```python
from build123d import *

# Parameters (mm, degrees)
SKETCH1_W           = 30
SKETCH1_H           = 19.61
SKETCH1_R           = 2.25
BOSS_EXTRUDE1_DEPTH = 7
SKETCH2_R           = 3.6
CUT_EXTRUDE1_DEPTH  = 2.8
FILLET2_R           = 5
BOSS_EXTRUDE2_DEPTH = 30


with BuildPart() as part:
    # Sketch1 → Boss-Extrude1 (new body)
    with BuildSketch(Plane.XY):
        Rectangle(SKETCH1_W, SKETCH1_H)
        with Locations((-10, -3.805)):
            Circle(SKETCH1_R, mode=Mode.SUBTRACT)
        with Locations((10, -3.805)):
            Circle(SKETCH1_R, mode=Mode.SUBTRACT)
    extrude(amount=BOSS_EXTRUDE1_DEPTH)

    # Sketch2 → Cut-Extrude1 (cut)
    with BuildSketch(Plane.XY.offset(7)):
        with Locations((-10, -3.805)):
            Circle(SKETCH2_R)
        with Locations((10, -3.805)):
            Circle(SKETCH2_R)
    extrude(amount=-CUT_EXTRUDE1_DEPTH, mode=Mode.SUBTRACT)

    # Fillet2
    fillet2_edges = [part.edges().sort_by_distance(p)[0] for p in [
        (15, -9.805, 3.5),
        (-15, -9.805, 3.5),
    ]]
    fillet(fillet2_edges, radius=FILLET2_R)

    # Sketch3 → Boss-Extrude2 (add, through all)
    with BuildSketch(Plane.ZY.offset(15)):
        Polygon((7, 1.805), (7, 9.805), (19, 9.805), (19, 6.805), align=None)
    extrude(amount=-BOSS_EXTRUDE2_DEPTH)


solid = part.part
```
Part model, mm, in its own coordinate system. A direction names the side the tool comes from. Round coordinates to 2 decimals unless told otherwise and drop trailing zeros. Loops run counter-clockwise (first coordinate to the right, second up) from the corner with the lowest first, then second, coordinate; pieces in that order, holes last.
Item 1: Cut at D-D, the plane x = 4.5. Give the cut face in (y, z) (3 decimals).
Item 2: Cut at A-A, the plane x = 9. Give the cut face in (y, z) (3 decimals), then the cut area to 3 significant figures.
Item 3: Cut at C-C, the plane y = -2.75. Give the cut face in (x, z), then the cut area to 3 significant figures.
Item 4: 3-axis set-ups, long thin cutter, end or side, ignore diameter. For faces 1 (the face through (12, -2, 4.2)), 2 (the face through (0, 8, 19)), 3 (the face through (0, -4, 7)): which of +Z, -Z, +X, -X, +Y, -Y reach the whole face in a straight line?
Item 5: Drill centre lines: line 1 (X direction, y = -4, z = 5.25); line 2 (Y direction, x = 10, z = 5.4) (3 decimals); line 3 (Y direction, x = -10, z = 3.35) (3 decimals). Where is each one in solid material? Low to high.
Item 6: Mould opens along X. For faces 4 (the face through (-6.566, -2.724, 5.62)), 5 (the face through (-13.574, -8.301, 3.549)), 6 (the face through (0, -9.805, 3)), 7 (the face through (13.434, -2.724, 5.62)) say: +X half, -X half, draft (parallel to the pull), parting line (faces both ways), or undercut.
Item 7: Cut at B-B, the plane z = 6.25. Give the cut face in (x, y) (3 decimals), then the cut area to 3 significant figures.
Item 8: Drop flat-ended pins along their axis: P1, Ø6, axis at x = -5, y = -6, coming from the +Z side; P2, Ø4, axis at x = -7, z = 11, coming from the -Y side; P3, Ø3.5, axis at x = 9.5, y = -3, coming from the +Z side. Give the stop position or say it passes through.
A:
1. outline: (-9.805, 0) - (9.805, 0) - (9.805, 19) - (6.805, 19) - (1.805, 7) - (-9.805, 7) - close
2. outline: (-9.805, 0) - (-5.821, 0) - (-5.821, 4.2) - (-7.263, 4.2) - (-7.263, 7) - (-9.805, 7) - close; (-1.789, 0) - (9.805, 0) - (9.805, 19) - (6.805, 19) - (1.805, 7) - (-0.347, 7) - (-0.347, 4.2) - (-1.789, 4.2) - close
2. area: 167 mm2
3. outline: (-15, 0) - (-11.99, 0) - (-11.99, 4.2) - (-13.44, 4.2) - (-13.44, 7) - (-15, 7) - close; (-8.01, 0) - (8.01, 0) - (8.01, 4.2) - (6.56, 4.2) - (6.56, 7) - (-6.56, 7) - (-6.56, 4.2) - (-8.01, 4.2) - close; (11.99, 0) - (15, 0) - (15, 7) - (13.44, 7) - (13.44, 4.2) - (11.99, 4.2) - close
3. area: 138 mm2
4. face 1: +Z
4. face 2: +Z, +X, -X, +Y, -Y
4. face 3: +Z, +X, -X, -Y
5. line 1: x = -15 to -13.59, -6.41 to 6.41, 13.59 to 15
5. line 2: y = -9.805 to -7.405, -0.205 to 9.805
5. line 3: y = -9.805 to -6.055, -1.555 to 9.805
6. face 4: undercut
6. face 5: -X half
6. face 6: draft
6. face 7: undercut
7. outline: (-15, -4.805) arc R5 ccw to (-10, -9.805) - (10, -9.805) arc R5 ccw to (15, -4.805) - (15, 9.805) - (-15, 9.805) - close; hole circle Ø7.2 at (-10, -3.805); hole circle Ø7.2 at (10, -3.805)
7. area: 496 mm2
8. P1: stops at z = 7
8. P2: stops at y = 2.64
8. P3: stops at z = 4.2
